Read the model definition and answer for the solid it produces. Units are mm, in the model's axes. A direction names the side the tool comes from. Coordinates: 2 decimals unless noted, no trailing zeros. Order: outer loops, then holes, each group sorted by start corner. A loop starts at its lowest first (then second) coordinate and runs counter-clockwise, first axis right, second up.
```python
from build123d import *

# Parameters (mm, degrees)
SKETCH1_W                 = 85.355339059
SKETCH1_H                 = 80.710678118
BOSS_EXTRUDE1_DEPTH       = 6.35
CUT_EXTRUDE1_DEPTH        = 0.5
CUT_EXTRUDE2_DEPTH        = 3.85
SKETCH4_W                 = 68
SKETCH4_H                 = 0.5
CUT_EXTRUDE3_DEPTH        = 1
SKETCH5_W                 = 68
SKETCH5_H                 = 0.5
CUT_EXTRUDE4_DEPTH        = 1
CUT_EXTRUDE5_DEPTH        = 7.35
SKETCH7_W                 = 30
SKETCH7_H                 = 9.355339059
CUT_EXTRUDE6_DEPTH        = 7.35
SKETCH8_W                 = 15.355339059
SKETCH8_H                 = 18
CUT_EXTRUDE7_DEPTH        = 7.35
CUT_EXTRUDE8_DEPTH        = 7.35
SKETCH10_W                = 30
SKETCH10_H                = 9.355339059
CUT_EXTRUDE9_DEPTH        = 7.35
CUT_EXTRUDE10_DEPTH       = 6.85
CUT_EXTRUDE11_DEPTH       = 1.5
DRAFT1_ANGLE              = 45
DRAFT2_ANGLE              = 45
DRAFT3_ANGLE              = 45
SKETCH13_W                = 10
SKETCH13_H                = 5.85
SKETCH14_W                = 2.5
SKETCH14_H                = 4.35
SKETCH15_W                = 2.5
SKETCH15_H                = 4.35
SKETCH16_W                = 2.5
SKETCH16_H                = 4.35
SKETCH17_W                = 2.5
SKETCH17_H                = 0.5
F_2_CLEARANCE_HOLE1_D     = 2.5
F_2_CLEARANCE_HOLE1_DEPTH = 6.35
F_3_CLEARANCE_HOLE1_D     = 3
F_3_CLEARANCE_HOLE1_DEPTH = 6.35
F_3_CLEARANCE_HOLE2_D     = 3
F_3_CLEARANCE_HOLE2_DEPTH = 6.35
F_3_CLEARANCE_HOLE3_D     = 3
F_3_CLEARANCE_HOLE3_DEPTH = 12
F_3_CLEARANCE_HOLE4_D     = 3
F_3_CLEARANCE_HOLE4_DEPTH = 12
F_3_CLEARANCE_HOLE5_D     = 3
F_3_CLEARANCE_HOLE5_DEPTH = 8
FILLET1_R                 = 3.175
FILLET2_R                 = 4.175
FILLET3_R                 = 5
FILLET4_R                 = 10


with BuildPart() as part:
    # Sketch1 → Boss-Extrude1 (new body)
    with BuildSketch(Plane.XY.offset(6.35)):
        with Locations((58.00266953, 0)):
            Rectangle(SKETCH1_W, SKETCH1_H)
    extrude(amount=-BOSS_EXTRUDE1_DEPTH)

    # Sketch2 → Cut-Extrude1 (cut)
    with BuildSketch(Plane.XY.offset(6.35)):
        with BuildLine():
            Line((15.325, -28), (83.325, -28))
            Line((83.325, -28), (83.325, -3.784507895))
            ThreePointArc((83.325, -3.784507895), (84.175, 0), (83.325, 3.784507894))
            Line((83.325, 3.784507894), (83.325, 28))
            Line((83.325, 28), (15.325, 28))
            Line((15.325, 28), (15.325, -28))
        make_face()
    extrude(amount=-CUT_EXTRUDE1_DEPTH, mode=Mode.SUBTRACT)

    # Sketch3 → Cut-Extrude2 (cut)
    with BuildSketch(Plane.XY.offset(5.85)):
        with BuildLine():
            Line((82.325, 5.415025392), (82.325, 28))
            Line((82.325, 28), (45.825, 28))
            Line((45.825, 28), (45.825, 10.874857598))
            ThreePointArc((45.825, 10.874857598), (46.581622253, 8.817657055), (48.490873433, 7.740943889))
            ThreePointArc((48.490873433, 7.740943889), (50.727145491, 6.201837814), (50.956306919, 3.4967971))
            ThreePointArc((50.956306919, 3.4967971), (69.866260129, 2.994053299), (54.63385571, -8.222583333))
            ThreePointArc((54.63385571, -8.222583333), (51.477391425, -14.794275673), (54.325, -21.505574533))
            Line((54.325, -21.505574533), (54.325, -28))
            Line((54.325, -28), (82.325, -28))
            Line((82.325, -28), (82.325, -5.415025392))
            ThreePointArc((82.325, -5.415025392), (84.175, 0), (82.325, 5.415025392))
        make_face()
    extrude(amount=-CUT_EXTRUDE2_DEPTH, mode=Mode.SUBTRACT)

    # Sketch4 → Cut-Extrude3 (cut)
    with BuildSketch(Plane.XZ.offset(-28)):
        with Locations((49.325, 6.1)):
            Rectangle(SKETCH4_W, SKETCH4_H)
    extrude(amount=-CUT_EXTRUDE3_DEPTH, mode=Mode.SUBTRACT)

    # Sketch5 → Cut-Extrude4 (cut)
    with BuildSketch(Plane(origin=(0, -28, 0), x_dir=(-1, 0, 0), z_dir=(0, 1, 0))):
        with Locations((-49.325, 6.1)):
            Rectangle(SKETCH5_W, SKETCH5_H)
    extrude(amount=-CUT_EXTRUDE4_DEPTH, mode=Mode.SUBTRACT)

    # Sketch6 → Cut-Extrude5 (cut, through all)
    with BuildSketch(Plane.XY.offset(6.35)):
        with BuildLine():
            Line((20.643770546, 40.355339059), (15.325, 40.355339059))
            Line((15.325, 40.355339059), (15.325, 31))
            ThreePointArc((15.325, 31), (19.350148184, 34.901195315), (20.643770546, 40.355339059))
        make_face()
    extrude(amount=-CUT_EXTRUDE5_DEPTH, mode=Mode.SUBTRACT)

    # Sketch7 → Cut-Extrude6 (cut, through all)
    with BuildSketch(Plane.XY.offset(6.35)):
        with Locations((60.325, 35.67766953)):
            Rectangle(SKETCH7_W, SKETCH7_H)
    extrude(amount=-CUT_EXTRUDE6_DEPTH, mode=Mode.SUBTRACT)

    # Sketch8 → Cut-Extrude7 (cut, through all)
    with BuildSketch(Plane.XY.offset(6.35)):
        with Locations((93.002669529, 0)):
            Rectangle(SKETCH8_W, SKETCH8_H)
    extrude(amount=-CUT_EXTRUDE7_DEPTH, mode=Mode.SUBTRACT)

    # Sketch9 → Cut-Extrude8 (cut, through all)
    with BuildSketch(Plane.XY.offset(6.35)):
        with BuildLine():
            Line((15.325, -31), (15.325, -40.355339059))
            Line((15.325, -40.355339059), (20.643770546, -40.355339059))
            ThreePointArc((20.643770546, -40.355339059), (19.350148184, -34.901195315), (15.325, -31))
        make_face()
    extrude(amount=-CUT_EXTRUDE8_DEPTH, mode=Mode.SUBTRACT)

    # Sketch10 → Cut-Extrude9 (cut, through all)
    with BuildSketch(Plane.XY.offset(6.35)):
        with Locations((60.325, -35.67766953)):
            Rectangle(SKETCH10_W, SKETCH10_H)
    extrude(amount=-CUT_EXTRUDE9_DEPTH, mode=Mode.SUBTRACT)

    # Sketch11 → Cut-Extrude10 (cut, through all)
    with BuildSketch(Plane.XY.offset(5.85)):
        with BuildLine():
            Line((15.325, 10), (15.325, -10))
            ThreePointArc((15.325, -10), (21.325, 0), (15.325, 10))
        make_face()
    extrude(amount=-CUT_EXTRUDE10_DEPTH, mode=Mode.SUBTRACT)

    # Sketch12 → Cut-Extrude11 (cut)
    with BuildSketch(Plane.XY.offset(5.85)):
        with BuildLine():
            Line((32.150000014, 12.5), (32.150000014, -10))
            ThreePointArc((32.150000014, -10), (35.325000015, -13.175000001), (38.500000016, -10))
            Line((38.500000016, -10), (38.500000016, 12.5))
            ThreePointArc((38.500000016, 12.5), (35.325000015, 15.675000001), (32.150000014, 12.5))
        make_face()
    extrude(amount=-CUT_EXTRUDE11_DEPTH, mode=Mode.SUBTRACT)

    # Draft1
    draft1_faces = [part.faces().sort_by_distance(p)[0] for p in [
        (45.325, 35.677669529, 3.175),
        (75.325, 35.677669529, 3.175),
    ]]
    draft(draft1_faces, Plane(origin=(45.325, 31, 0), x_dir=(1, 0, 0), z_dir=(0, 1, 0)), DRAFT1_ANGLE)

    # Draft2
    draft2_faces = [part.faces().sort_by_distance(p)[0] for p in [
        (45.325, -35.67766953, 3.175),
        (75.325, -35.677669529, 3.175),
    ]]
    draft(draft2_faces, Plane(origin=(75.325, -31, 0), x_dir=(0, 0, -1), z_dir=(0, -1, 0)), DRAFT2_ANGLE)

    # Draft3
    draft3_faces = [part.faces().sort_by_distance(p)[0] for p in [
        (93.002669529, 9, 3.175),
        (93.002669529, -9, 3.175),
    ]]
    draft(draft3_faces, Plane(origin=(85.325, 9, 0), x_dir=(0, 0, 1), z_dir=(1, 0, 0)), DRAFT3_ANGLE)

    # Sketch13 → Cut-Revolve1 (revolve, cut)
    with BuildSketch(Plane.XZ):
        with Locations((65.325, 2.925)):
            Rectangle(SKETCH13_W, SKETCH13_H)
    revolve(axis=Axis((60.325, 0, 5.85), (0, 0, -1)), mode=Mode.SUBTRACT)

    # Sketch14 → Revolve1 (revolve)
    with BuildSketch(Plane.XZ.offset(-15)):
        with Locations((61.575, 4.175)):
            Rectangle(SKETCH14_W, SKETCH14_H)
    revolve(axis=Axis((60.325, 15, 6.35), (0, 0, -1)))

    # Sketch15 → Revolve2 (revolve)
    with BuildSketch(Plane.XZ):
        with Locations((76.575, 4.175)):
            Rectangle(SKETCH15_W, SKETCH15_H)
    revolve(axis=Axis((75.325, 0, 6.35), (0, 0, -1)))

    # Sketch16 → Revolve3 (revolve)
    with BuildSketch(Plane.XZ.offset(15)):
        with Locations((61.575, 4.175)):
            Rectangle(SKETCH16_W, SKETCH16_H)
    revolve(axis=Axis((60.325, -15, 6.35), (0, 0, -1)))

    # Sketch17 → Revolve4 (revolve)
    with BuildSketch(Plane(origin=(0, 0, 0), x_dir=(1, 0, 0), z_dir=(0, 1, 0))):
        with Locations((46.575, -6.1)):
            Rectangle(SKETCH17_W, SKETCH17_H)
    revolve(axis=Axis((45.325, 0, 5.85), (0, 0, 1)))

    # #2 Clearance Hole1
    with Locations(Plane(origin=(0, 0, 0), x_dir=(-1, 0, 0), z_dir=(0, 0, -1))):
        with Locations((-22.325, -24), (-22.325, 24)):
            Hole(F_2_CLEARANCE_HOLE1_D / 2, depth=F_2_CLEARANCE_HOLE1_DEPTH)

    # #3 Clearance Hole1
    with Locations(Plane.XY.offset(6.35)):
        with Locations((45.325, 0), (60.325, 15), (75.325, 0), (60.325, -15)):
            Hole(F_3_CLEARANCE_HOLE1_D / 2, depth=F_3_CLEARANCE_HOLE1_DEPTH)

    # #3 Clearance Hole2
    with Locations(Plane(origin=(0, 0, 0), x_dir=(-1, 0, 0), z_dir=(0, 0, -1))):
        with Locations((-24.969660941, 35.355339059), (-95.680339059, 35.355339059), (-95.680339059, -35.355339059), (-24.969660941, -35.355339059)):
            Hole(F_3_CLEARANCE_HOLE2_D / 2, depth=F_3_CLEARANCE_HOLE2_DEPTH)

    # #3 Clearance Hole3
    with Locations(Plane(origin=(0, -40.355339059, 0), x_dir=(-1, 0, 0), z_dir=(0, -1, 0))):
        with Locations((-30.325, -3.175), (-90.325, -3.175)):
            Hole(F_3_CLEARANCE_HOLE3_D / 2, depth=F_3_CLEARANCE_HOLE3_DEPTH)

    # #3 Clearance Hole4
    with Locations(Plane(origin=(0, 40.355339059, 0), x_dir=(1, 0, 0), z_dir=(0, 1, 0))):
        with Locations((90.325, -3.175), (30.325, -3.175)):
            Hole(F_3_CLEARANCE_HOLE4_D / 2, depth=F_3_CLEARANCE_HOLE4_DEPTH)

    # #3 Clearance Hole5
    with Locations(Plane(origin=(100.680339059, 0, 0), x_dir=(0, 0, -1), z_dir=(1, 0, 0))):
        with Locations((-3.175, -30), (-3.175, 30)):
            Hole(F_3_CLEARANCE_HOLE5_D / 2, depth=F_3_CLEARANCE_HOLE5_DEPTH)

    # Fillet1
    fillet1_edges = [part.edges().sort_by_distance(p)[0] for p in [
        (82.325, 5.415025392, 3.925),
        (82.325, -5.415025392, 3.925),
        (82.325, -28, 3.925),
        (54.325, -28, 3.925),
        (54.325, -21.505574533, 3.925),
        (54.63385571, -8.222583333, 3.925),
        (45.825, 28, 3.925),
        (82.325, 28, 3.925),
    ]]
    fillet(fillet1_edges, radius=FILLET1_R)

    # Fillet2
    fillet2_edges = [part.edges().sort_by_distance(p)[0] for p in [
        (83.325, 29, 6.1),
        (83.325, -29, 6.1),
    ]]
    fillet(fillet2_edges, radius=FILLET2_R)

    # Fillet3
    fillet3_edges = [part.edges().sort_by_distance(p)[0] for p in [
        (35.969660941, -40.355339059, 3.175),
        (84.680339059, 40.355339059, 3.175),
        (100.680339059, 40.355339059, 3.175),
        (100.680339059, -24.355339059, 3.175),
        (15.325, 10, 2.925),
        (15.325, -10, 2.925),
        (100.680339059, 24.355339059, 3.175),
        (100.680339059, -40.355339059, 3.175),
        (35.969660941, 40.355339059, 3.175),
        (84.680339059, -40.355339059, 3.175),
        (20.643770546, 40.355339059, 3.175),
        (15.325, 31, 3.175),
        (15.325, -31, 3.175),
        (20.643770546, -40.355339059, 3.175),
    ]]
    fillet(fillet3_edges, radius=FILLET3_R)

    # Fillet4
    fillet4_edges = [part.edges().sort_by_distance(p)[0] for p in [
        (75.325, 31, 3.175),
        (45.325, 31, 3.175),
        (85.325, -9, 3.175),
        (85.325, 9, 3.175),
        (45.325, -31, 3.175),
        (75.325, -31, 3.175),
    ]]
    fillet(fillet4_edges, radius=FILLET4_R)


solid = part.part
```
1) A cutting plane is placed at A-A, the plane x = 67. Determine the outline of the cut face in (y, z).
A:
outline: (-31, 0) - (-7.45, 0) - (-7.45, 2) - (-28, 2) - (-28, 5.85) - (-29, 5.85) - (-29, 6.35) - (-31, 6.35) - close; (7.45, 0) - (31, 0) - (31, 6.35) - (29, 6.35) - (29, 5.85) - (28, 5.85) - (28, 2) - (7.45, 2) - close
2) Straight lines are drawn through the part: line 1 (Y direction, x = 25.5, z = 4); line 2 (X direction, y = 34.5, z = 3.5) (3 decimals); line 3 (Y direction, x = 70, z = 6). For each, find the intervals that lie inside material, in ascending order.
A:
line 1: y = -40.36 to -36.76, -33.95 to 33.95, 36.76 to 40.36
line 2: x = 19.109 to 23.737, 26.202 to 28.861, 31.789 to 41.825, 78.825 to 88.861, 91.789 to 94.448, 96.913 to 100.68
line 3: y = -31 to -29, 29 to 31
3) A cutting plane is placed at C-C, the plane y = -30. Determine the outline of the cut face in (x, z) (3 decimals).
A:
outline: (15.596, 0) - (100.68, 0) - (100.68, 1.675) - (92.68, 1.675) - (92.68, 4.675) - (100.68, 4.675) - (100.68, 6.35) - (15.596, 6.35) - close; hole circle Ø3 at (30.325, 3.175); hole circle Ø3 at (90.325, 3.175)
4) Which of the six approach directions +Z, -Z, +X, -X, +Y, -Y give full straight-line access (tool end or side, diameter ignored) to faces 5 (the cylindrical face through (35.787, 39.985, 3.131)), 6 (the cylindrical face through (84.813, -39.964, 3.131)), 7 (the flat face through (35, 1, 4.35))?
A:
face 5: +Z, -Z, +Y
face 6: +Z, -Z, -Y
face 7: +Z
5) A cutting plane is placed at B-B, the plane y = -15. Determine the outline of the cut face in (x, z) (3 decimals), and give its area (3 significant figures).
A:
outline: (15.325, 0) - (58.825, 0) - (58.825, 6.35) - (57.825, 6.35) - (57.825, 2) - (51.475, 2) - (51.475, 5.85) - (15.325, 5.85) - close; (61.825, 0) - (91.325, 0) - (91.325, 6.35) - (83.325, 6.35) - (83.325, 5.85) - (82.325, 5.85) - (82.325, 2) - (62.825, 2) - (62.825, 6.35) - (61.825, 6.35) - close
area: 333 mm2
6) Determine the mould class of faces 1 (the cylindrical face through (96.624, 31.487, 2.98)), 2 (the cylindrical face through (54.136, -21.695, 3.898)), 3 (the flat face through (15.325, 20, 3)), 4 (the cylindrical face through (19.004, -34.337, 3.219)) for opening direction Y: pulls with the +Y half, pulls with the -Y half, needs draft (parallel to the pull), parting line crosses it, or undercut.
A:
face 1: undercut
face 2: undercut
face 3: needs draft
face 4: pulls with the -Y half
7) Flat-ended cylindrical pins translate along their axes: pin 1 Ø2.5 at (x, y) = (24.97, 35.36) entering from +Z (1 decimal); pin 2 Ø1 at (y, z) = (-17.5, 3) entering from +X (3 decimals); pin 3 Ø0.9 at (x, z) = (90, 3.5) entering from -Y; pin 4 Ø3 at (x, z) = (62.5, 4.5) entering from -Y. Find the tip coordinate at first contact, or state that the pin passes through.
A:
pin 1: passes through
pin 2: stops at x = 94.325
pin 3: stops at y = -28.36
pin 4: stops at y = -31
